Part model, mm, in its own coordinate system. A direction names the side the tool comes from. Round coordinates to 2 decimals unless told otherwise and drop trailing zeros. Loops run counter-clockwise (first coordinate to the right, second up) from the corner with the lowest first, then second, coordinate; pieces in that order, holes last. Notation, with made-up numbers: (20.25, 44.25) - (77.25, 44.25) arc R15 ccw to (77.25, 70.25) - close; hole circle Ø6 at (-12.75, -32.75). An arc over 180 degrees is marked (long way). Put each result on its own line as item: value.
from build123d import *

# Parameters (mm, degrees)
SKETCH_1_W                              = 20
SKETCH_1_H                              = 20
BASEBOX_DEPTH                           = 10
HOLE_BLINDCBORE_THRU_DEPTH8_D           = 6
HOLE_BLINDCBORE_THRU_DEPTH8_DEPTH       = 8
HOLE_BLINDCBORE_THRU_DEPTH8_CBORE_D     = 11
HOLE_BLINDCBORE_THRU_DEPTH8_CBORE_DEPTH = 6


with BuildPart() as part:
    # 草图1 → BaseBox (new body)
    with BuildSketch(Plane.XY):
        with Locations((10, 10)):
            Rectangle(SKETCH_1_W, SKETCH_1_H)
    extrude(amount=BASEBOX_DEPTH)

    # Hole_BlindCbore_thru_depth8
    with Locations(Plane.XY.offset(10)):
        with Locations((9.986487375, 10.014305599)):
            CounterBoreHole(HOLE_BLINDCBORE_THRU_DEPTH8_D / 2, HOLE_BLINDCBORE_THRU_DEPTH8_CBORE_D / 2, HOLE_BLINDCBORE_THRU_DEPTH8_CBORE_DEPTH, depth=HOLE_BLINDCBORE_THRU_DEPTH8_DEPTH)


solid = part.part
1. Tool access for faces 5 (the flat face through (12.4, 7.6, 4)), 6 (the flat face through (10, 20, 5)): list every direction of +Z, -Z, +X, -X, +Y, -Y with a clear straight run to the whole face (end or side of a thin tool).
A:
face 5: +Z
face 6: +Z, -Z, +X, -X, +Y
2. Band-saw the part on A-A (z = 7). List the corners of the cut face in (x, y).
A:
outline: (0, 0) - (20, 0) - (20, 20) - (0, 20) - close; hole circle Ø11 at (9.99, 10.01)
3. Pin check, flat tip, straight feed: P1, Ø3, axis at x = 11, y = 10.5, coming from the +Z side. Stop position of the tip, or through.
A:
P1: stops at z = 2
4. Band-saw the part on B-B (x = 12.5). List the corners of the cut face in (y, z), plus the area to 3 significant figures.
A:
outline: (0, 0) - (20, 0) - (20, 10) - (14.91, 10) - (14.91, 4) - (11.65, 4) - (11.65, 2) - (8.38, 2) - (8.38, 4) - (5.12, 4) - (5.12, 10) - (0, 10) - close
area: 135 mm²
5. Probe line 1 along Z through (x, y) = (14.5, 11.75); line 2 along X through (y, z) = (11.5, 4.5); line 3 along Y through (x, z) = (7.5, 7.75). List the from-to ranges inside material, lowest first. Write a range as [from, to].
A:
line 1: z = [0, 4]
line 2: x = [0, 4.69], [15.28, 20]
line 3: y = [0, 5.11], [14.92, 20]
6. Band-saw the part on C-C (y = 6). List the corners of the cut face in (x, z).
A:
outline: (0, 0) - (20, 0) - (20, 10) - (13.75, 10) - (13.75, 4) - (6.23, 4) - (6.23, 10) - (0, 10) - close
7. Two-plate mould, pull along X, no slides. Class faces 1 (the flat face through (0, 10, 5)), 2 (the flat face through (20, 10, 5)), 3 (the flat face through (10, 10, 2)), 4 (the cylindrical face through (10.38, 12.99, 2.99)): pulls with the +X half, pulls with the -X half, needs draft (parallel to the pull), parting line crosses it, or undercut.
A:
face 1: pulls with the -X half
face 2: pulls with the +X half
face 3: undercut
face 4: undercut
8. Band-saw the part on D-D (z = 2.25). List the corners of the cut face in (x, y), plus the area to 3 significant figures.
A:
outline: (0, 0) - (20, 0) - (20, 20) - (0, 20) - close; hole circle Ø6 at (9.99, 10.01)
area: 372 mm²
